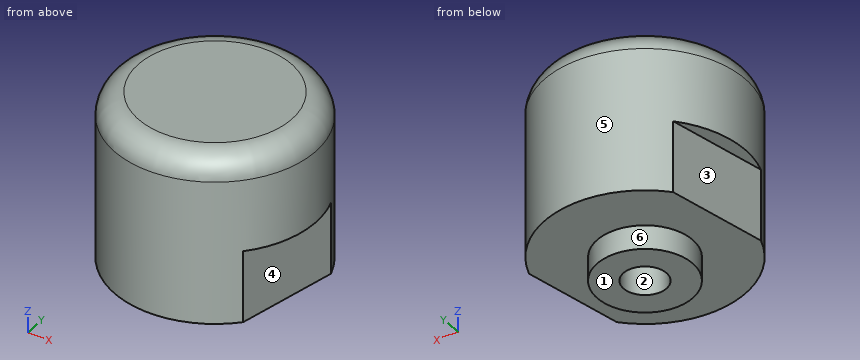
```python
from build123d import *

# Parameters (mm, degrees)
SKETCH1_R           = 21
BOSS_EXTRUDE1_DEPTH = 40
SKETCH2_R           = 21
SKETCH2_R_2         = 10
CUT_EXTRUDE1_DEPTH  = 5
CUT_EXTRUDE2_DEPTH  = 15
FILLET1_R           = 5
SKETCH3_R           = 4.5
CUT_EXTRUDE3_DEPTH  = 10


with BuildPart() as part:
    # Sketch1 → Boss-Extrude1 (new body)
    with BuildSketch(Plane.XY):
        Circle(SKETCH1_R)
    extrude(amount=BOSS_EXTRUDE1_DEPTH)

    # Sketch2 → Cut-Extrude1 (cut)
    with BuildSketch(Plane(origin=(0, 0, 0), x_dir=(-1, 0, 0), z_dir=(0, 0, -1))):
        Circle(SKETCH2_R)
        Circle(SKETCH2_R_2, mode=Mode.SUBTRACT)
    extrude(amount=-CUT_EXTRUDE1_DEPTH, mode=Mode.SUBTRACT)

    # Sketch4 → Cut-Extrude2 (cut)
    with BuildSketch(Plane(origin=(0, 0, 5), x_dir=(-1, 0, 0), z_dir=(0, 0, -1))):
        with BuildLine():
            Line((15.379257562, 14.299595688), (19.84526591, -6.867708567))
            ThreePointArc((19.84526591, -6.867708567), (20.547638692, 4.335267488), (15.379257562, 14.299595688))
        make_face()
    cut_extrude2 = extrude(amount=-CUT_EXTRUDE2_DEPTH, mode=Mode.SUBTRACT)

    # Mirror1: Cut-Extrude2 across plane
    add(cut_extrude2.mirror(Plane(origin=(0, 0, 0), x_dir=(0, 0, 1), z_dir=(-0.9784589853258884, 0.20644130893557386, 0))), mode=Mode.SUBTRACT)

    # Fillet1
    fillet1_edges = [part.edges().sort_by_distance(p)[0] for p in [
        (-21, 0, 40),
    ]]
    fillet(fillet1_edges, radius=FILLET1_R)

    # Sketch3 → Cut-Extrude3 (cut)
    with BuildSketch(Plane(origin=(0, 0, 0), x_dir=(-1, 0, 0), z_dir=(0, 0, -1))):
        Circle(SKETCH3_R)
    extrude(amount=-CUT_EXTRUDE3_DEPTH, mode=Mode.SUBTRACT)


solid = part.part
```
Here's how the part is built. I have some questions about the finished solid (model axes, mm). Face numbers are marked on the shaded views. A direction names the side the tool comes from. Give positions to 0.01 mm unless a question says otherwise; leave off trailing zeros. Order: outer loops, then holes, each group sorted by start corner. A loop starts at its lowest first (then second) coordinate and runs counter-clockwise, first axis right, second up. Notation, with made-up numbers: (66.25, 60.5) -> (125.25, 60.5) arc R21 cw to (125.25, 96.5) -> close; hole circle Ø1 at (67, 78). An arc over 180 degrees is marked (long way). Use CSV: the item, a comma, the result in double quotes. Start each with the question number.
Item 1: On a 3-axis mill with a long thin cutter (end or side, diameter ignored), from which of +Z, -Z, +X, -X, +Y, -Y can I reach the whole of each face in a straight line? I mean the marked faces 5 and 6. Say none if no direction works.
Item 2: Suppose I cut it at C-C (y = 0). List the corners of the cut face in (x, z) for me, and give its area (3 significant figures).
Item 3: Thinking about a two-plate mould opening in Y: for the marked faces 1, 2, 3 and 4, which applies, pulls with the +Y half, pulls with the -Y half, needs draft (parallel to the pull), parting line crosses it, or undercut?
Item 4: I'm going to push flat-ended pins straight in: P1, Ø12, axis at x = -8.5, z = 26.5, coming from the +Y side; P2, Ø5, axis at y = -10, z = 16.5, coming from the -X side; P3, Ø5.5, axis at x = 0, y = 0, coming from the -Z side. Where does each tip first touch, or does it pass through?
Item 5: If I drill on probe 1 along Y at (x, z) = (0, 4); probe 2 along Y at (x, z) = (0, 5.75); probe 3 along Z at (x, y) = (9, -11), over which ranges is the centre line in solid material (lowest first)? Write a range as [from, to].
Item 6: Suppose I cut it at B-B (z = 26). List the corners of the cut face in (x, y) for me, and give its area (3 significant figures).
Item 7: Suppose I cut it at D-D (z = 19). List the corners of the cut face in (x, y) for me.
Item 8: Suppose I cut it at A-A (x = 0). List the corners of the cut face in (y, z) for me, and give its area (3 significant figures).
Answer block:
1,face 5,"+Z, -Z"
1,face 6,"-Z"
2,outline,"(-21, 20) -> (-18.4, 20) -> (-18.4, 5) -> (-10, 5) -> (-10, 0) -> (-4.5, 0) -> (-4.5, 10) -> (4.5, 10) -> (4.5, 0) -> (10, 0) -> (10, 5) -> (18.4, 5) -> (18.4, 20) -> (21, 20) -> (21, 35) arc R5 ccw to (16, 40) -> (-16, 40) arc R5 ccw to (-21, 35) -> close"
2,area,"1,390 mm^2"
3,face 1,"needs draft"
3,face 2,"undercut"
3,face 3,"pulls with the +Y half"
3,face 4,"pulls with the -Y half"
4,P1,"stops at y = 20.85"
4,P2,"stops at x = -19.62"
4,P3,"stops at z = 10"
5,probe 1,"y = [-10, -4.5], [4.5, 10]"
5,probe 2,"y = [-21, -4.5], [4.5, 21]"
5,probe 3,"z = [5, 40]"
6,outline,"circle Ø42 at (0, 0)"
6,area,"1,390 mm^2"
7,outline,"(-19.85, -6.87) arc R21 ccw to (15.38, -14.3) -> (19.85, 6.87) arc R21 ccw to (-15.38, 14.3) -> close"
8,outline,"(-21, 5) -> (-10, 5) -> (-10, 0) -> (-4.5, 0) -> (-4.5, 10) -> (4.5, 10) -> (4.5, 0) -> (10, 0) -> (10, 5) -> (21, 5) -> (21, 35) arc R5 ccw to (16, 40) -> (-16, 40) arc R5 ccw to (-21, 35) -> close"
8,area,"1,470 mm^2"
